Autodesk Inventor part; units mm, degrees
ref_plane "YZ Plane" through (0, 0, 0) normal (1, 0, 0) x (0, 1, 0)
ref_plane "XZ Plane" through (0, 0, 0) normal (0, 1, 0) x (-1, 0, 0)
ref_plane "XY Plane" through (0, 0, 0) normal (0, 0, 1) x (1, 0, 0)
sketch "Sketch1" plane through (0, 0, 0) normal (0, 0, 1) x (1, 0, 0)
  circle A0 centre (0, 0) radius 0.762
  line L0 (-1.0776, 0) -> (0, 1.0776)
  line L1 (0, 1.0776) -> (1.0776, 0)
  line L2 (1.0776, 0) -> (0, -1.0776)
  line L3 (0, -1.0776) -> (-1.0776, 0)
  line L4 (-0.762, 0.762) -> (0.762, 0.762)
  line L5 (0.762, 0.762) -> (0.762, -0.762)
  line L6 (0.762, -0.762) -> (-0.762, -0.762)
  line L7 (-0.762, -0.762) -> (-0.762, 0.762)
  point P0 (0, 3.175)
  point P1 (-3.175, 0)
  point P2 (-0.898, 0.898)
  point P3 (-0.6286, -0.0898)
  point P4 (-0.5388, -0.5388)
  point P5 (0.5388, -0.5388)
  point P6 (0.3287, 1.2267)
  point P7 (3.7343, 0.7559)
  point P8 (0.5388, 0.5388)
  point P9 (-0.5388, 0.5388)
  point P10 (0, 0.762)
  point P11 (-0.762, 0)
  point P12 (0.3156, 0.762)
  point P13 (-0.3156, 0.762)
  point P14 (-0.762, 0.3156)
  point P15 (-0.762, -0.3156)
  point P16 (-0.3156, -0.762)
  point P17 (0.3156, -0.762)
  point P18 (0.762, -0.3156)
  point P19 (0.762, 0.3156)
  dimension "d0" = 1.524
  dimension "d1" = 1.524
  dimension "d2" = 1.524
  dimension "d3" = 0
  dimension "d12" = 0
  dimension "d13" = 0
  dimension "d16" = 1.524
  dimension "d17" = 1.524
  dimension "d18" = 0
  dimension "d19" = 0
extrude "Extrusion3" add sketch "Sketch1" against normal blind 7.62
sketch "Sketch6" plane through (0, 0, 0) normal (0, 0, 1) x (1, 0, 0)
  line L0 (-0.762, 0.3156) -> (-0.762, 0.762)
  circle A0 centre (0, 0) radius 1.0776
  line L1 (-0.762, 0.762) -> (-0.3156, 0.762)
  circle A1 centre (0, 0) radius 0.635
  dimension "d33" = 1.27
extrude "Extrusion6" cut sketch "Sketch6" against normal blind 5.08
sketch "Sketch7" plane through (0, 0, -7.62) normal (0, 0, -1) x (-1, 0, 0)
  line L0 (-1.6188, 0.635) -> (1.6188, 0.635) construction
  line L1 (1.6188, 0.635) -> (1.6188, -0.635) construction
  line L2 (1.6188, -0.635) -> (-1.6188, -0.635) construction
  line L3 (-1.6188, -0.635) -> (-1.6188, 0.635) construction
  line L4 (-0.1528, -0.1398) -> (-0.1528, -0.2286)
  line L5 (-0.1528, -0.2286) -> (0.0123, -0.2286)
  line L6 (0.0123, -0.2286) -> (0.0123, 0.2282)
  line L7 (0.0123, 0.2282) -> (-0.1657, 0.2282)
  spline S0 degree 2 poles (-0.1657, 0.2282) (-0.2188, 0.2282) (-0.291, 0.1916) (-0.3147, 0.1563) knots 0 0 0 1 2 2 2
  line L8 (-0.3147, 0.1563) -> (-0.5796, -0.2286)
  line L9 (-0.5796, -0.2286) -> (-0.3825, -0.2286)
  line L10 (-0.3825, -0.2286) -> (-0.3258, -0.1398)
  line L11 (-0.3258, -0.1398) -> (-0.1528, -0.1398)
  line L12 (-0.25, -0.0203) -> (-0.1769, 0.0943)
  spline S1 degree 2 poles (-0.1769, 0.0943) (-0.1715, 0.1028) (-0.1608, 0.1091) (-0.1541, 0.1086) knots 0 0 0 1 2 2 2
  line L13 (-0.1541, 0.1086) -> (-0.1528, 0.1086)
  line L14 (-0.1528, 0.1086) -> (-0.1528, -0.0203)
  line L15 (-0.1528, -0.0203) -> (-0.25, -0.0203)
  line L16 (0.0783, 0.1086) -> (0.238, 0.1086)
  line L17 (0.238, 0.1086) -> (0.238, -0.2286)
  line L18 (0.238, -0.2286) -> (0.403, -0.2286)
  line L19 (0.403, -0.2286) -> (0.403, 0.1086)
  line L20 (0.403, 0.1086) -> (0.5627, 0.1086)
  line L21 (0.5627, 0.1086) -> (0.5627, 0.2282)
  line L22 (0.5627, 0.2282) -> (0.0801, 0.2282)
  line L23 (0.0801, 0.2282) -> (0.0783, 0.1086)
  point P0 (0, 0)
  point P1 (0, 0.635)
  point P2 (-1.6188, 0)
  dimension "d34" = 0
  dimension "d35" = 0
extrude "Extrusion7" cut sketch "Sketch7" against normal blind 0.508
properties part number "screwhead"
Build history of the part. All positions in model axes, mm. Round coordinates to 2 decimals unless told otherwise and drop trailing zeros. Write each loop counter-clockwise with the first axis right and the second up, starting at its lowest first coordinate (ties: lowest second). Pieces come first, ordered by that corner, then holes. Notation, with made-up numbers: M -24,-15 L 28,-15 A16 cw 28,15 Z; hole C 12,-34 d2. An arc over 180 degrees is marked long. Use CSV: the item, a comma, the result in double quotes.
1. Two-plate mould, pull along X, no slides. Class faces 1 (the face through (-0.08, 0.63, -2.5)), 2 (the face through (0, 0, 0)): +X half, -X half, draft (parallel to the pull), parting line (faces both ways), or undercut.
Reply:
face 1,"parting line"
face 2,"draft"
2. Saw through at A-A (z = -1). Give the cut face in (x, y) (3 decimals), plus the area to 3 significant figures.
Reply:
outline,"C 0,0 d1.27"
area,"1.27 mm²"
3. Flat gauge pins, fed straight in: pin 1 (1 mm diameter, centred on x = 0.5, z = -3.5, fed in from +Y) (3 decimals); pin 2 (0.5 mm diameter, centred on y = -0.5, z = -6.5, fed in from +X). Where does each tip first touch, or does it go through?
Reply:
pin 1,"stops at y = 0.635"
pin 2,"stops at x = 0.83"
4. Wall check: probe 1 along Z at (x, y) = (-0.35, 0.65); probe 2 along X at (y, z) = (0.65, -5.5); probe 3 along Y at (x, z) = (-0.55, -2). Give the ranges that are in metal, low to high. Write a range as from..to.
Reply:
probe 1,"z = -7.62..-5.08"
probe 2,"x = -0.76..0.76"
probe 3,"y = -0.32..0.32"
5. Saw through at B-B (x = -0.9). Give the cut face in (y, z), plus the area to 3 significant figures.
Reply:
outline,"M -0.18,-7.62 L 0.18,-7.62 L 0.18,-5.08 L -0.18,-5.08 Z"
area,"0.902 mm²"
